Geometry: see drawing. Coordinates: mm, zero at the bounding-box minimum. Give positions to 0.01 mm unless a question says otherwise; leave off trailing zeros. Loops run counter-clockwise (first coordinate to the right, second up) from the corner with the lowest first, then second, coordinate; pieces in that order, holes last. Notation, with made-up numbers: (-37, 19) -> (-33, 19) arc R29 cw to (-33, 48) -> close; hole circle Ø6 at (21, -28.75). An arc over 180 degrees is marked (long way). Return JSON: item names as keys, results as strings. Group by question number.
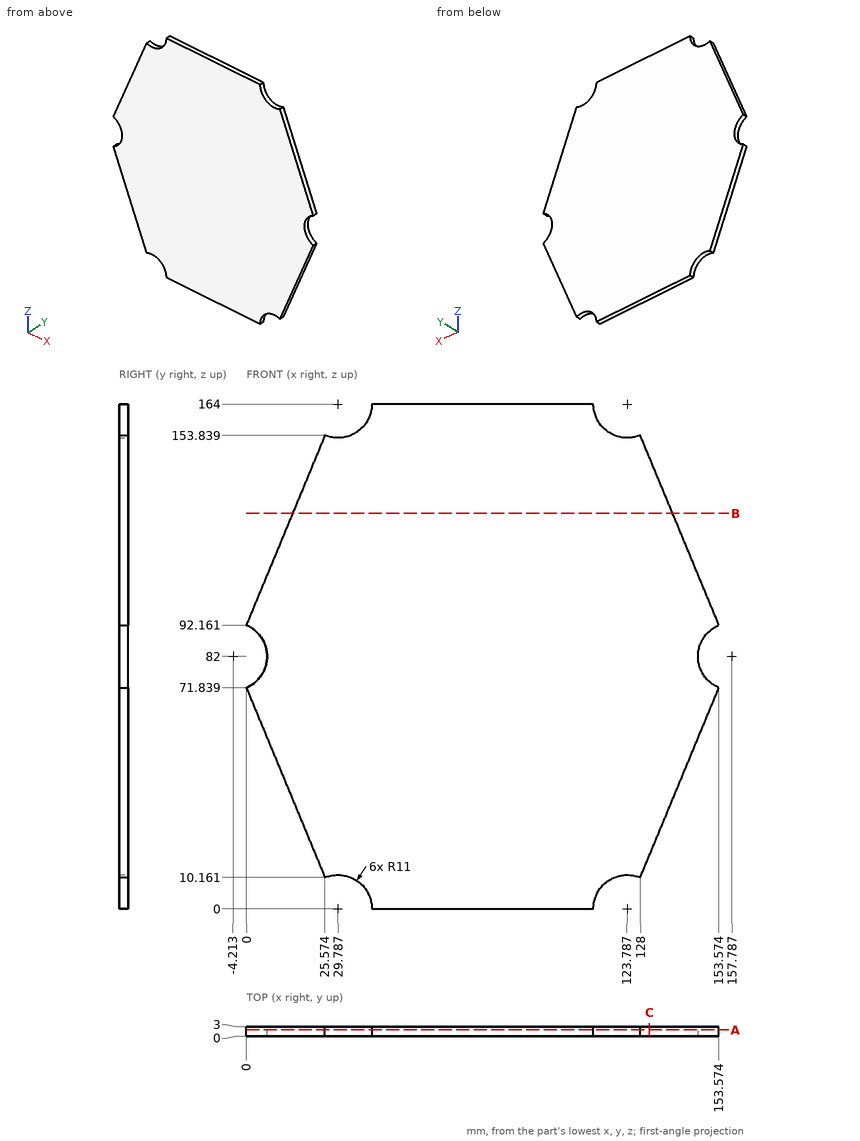
1) Contact query for a flat-ended pin moving along its axis: P1, Ø1, axis at y = 1.5, z = 129, coming from the -X side. Output: stop coordinate, or through.
2) Material intervals for line 1 (X direction, y = 1.1, z = 82.5) (1 decimal); line 2 (X direction, y = 2, z = 55); line 3 (Z direction, x = 115.5, y = 1.8) (1 decimal), sorted ascending.
3) Cut plane C-C on x = 131. Return loops of the section in (y, z).
4) Cut plane B-B on z = 128.5. Return loops of the section in (x, y), then the cut area to 3 significant figures.
5) Cut plane A-A on y = 1.95. Return loops of the section in (x, z).
Calculated:
{
 "1": {"P1": "x = 15.07"},
 "2": {"line 1": "6.8 to 146.8", "line 2": "6.98 to 146.59", "line 3": "7.2 to 156.8"},
 "3": {"outline": "(0, 17.4) -> (3, 17.4) -> (3, 146.6) -> (0, 146.6) -> close"},
 "4": {"outline": "(15.07, 0) -> (138.51, 0) -> (138.51, 3) -> (15.07, 3) -> close", "area": "370 mm2"},
 "5": {"outline": "(0, 71.84) -> (25.57, 10.16) arc R11 cw to (40.79, 0) -> (112.79, 0) arc R11 cw to (128, 10.16) -> (153.57, 71.84) arc R11 cw to (153.57, 92.16) -> (128, 153.84) arc R11 cw to (112.79, 164) -> (40.79, 164) arc R11 cw to (25.57, 153.84) -> (0, 92.16) arc R11 cw to start"}
}
